from build123d import *
from OCP.BRepFilletAPI import BRepFilletAPI_MakeChamfer

# Parameters (mm, degrees)
BOSS_EXTRUDE2_DEPTH       = 40
CHAMFER1_SIZE             = 15
CHAMFER3_SIZE             = 2.5
CHAMFER3_SIZE2            = 2.68451721
M4X0_7_TAPPED_HOLE1_D     = 3.3
M4X0_7_TAPPED_HOLE1_DEPTH = 10.1
M4X0_7_TAPPED_HOLE1_TIP   = 0.991420021
SKETCH4_R                 = 11.5
CUT_EXTRUDE1_DEPTH        = 30
M6X1_0_TAPPED_HOLE1_D     = 5
M6X1_0_TAPPED_HOLE1_DEPTH = 15
M6X1_0_TAPPED_HOLE1_TIP   = 1.502151548


with BuildPart() as part:
    # Sketch1 → Boss-Extrude2 (new body)
    with BuildSketch(Plane(origin=(0, 0, 0), x_dir=(1, 0, 0), z_dir=(0, 1, 0))):
        with BuildLine():
            Line((-28, 48), (-48, 48))
            Line((-48, 48), (-93, 45))
            Line((-93, 45), (-93, -45))
            Line((-93, -45), (-48, -48))
            Line((-48, -48), (-28, -48))
            Line((-28, -48), (-28, -38.987177379))
            ThreePointArc((-28, -38.987177379), (-48, 0), (-28, 38.987177379))
            Line((-28, 38.987177379), (-28, 48))
        make_face()
    extrude(amount=BOSS_EXTRUDE2_DEPTH)

    # Chamfer1
    chamfer1_edges = [part.edges().sort_by_distance(p)[0] for p in [
        (-48, 40, 0),
    ]]
    chamfer(chamfer1_edges, length=CHAMFER1_SIZE)

    # Chamfer2
    # the kernel refuses this chamfer: 2.5 mm, written as the material it takes off along each edge
    with BuildSketch(Plane(origin=(-32.604077303, 40, -49.026394846), x_dir=(0.06649386081081782, 0.027495876610587725, 0.9974079121622642), z_dir=(-0.997785157856609, 0, 0.06651901052377412)), Plane(origin=(-108.395922697, 40, 43.973605154), x_dir=(0.06649386081081746, 0.02749587661058773, -0.9974079121622642), z_dir=(0.997785157856609, 0, 0.06651901052377378))) as chamfer2_piece_1:
        with BuildLine():
            Line((2.571682988, 0), (-0.141367887, -2.567794484))
            Line((-0.141367887, -2.567794484), (-0.191348983, -2.56641969))
            ThreePointArc((-0.191348983, -2.56641969), (-0.085323068, -1.283494574), (-0.049981096, 0.001374794))
            Line((-0.049981096, 0.001374794), (0.001374794, 0.049981096))
            ThreePointArc((0.001374794, 0.049981096), (1.286244162, 0.014639124), (2.573057782, 0.049981096))
            Line((2.573057782, 0.049981096), (2.571682988, 0))
        make_face()
    extrude(amount=75.960084991, mode=Mode.SUBTRACT)
    with BuildSketch(Plane(origin=(-93, 40, -60.430097928), x_dir=(0.9996219169112968, 0.027495876610587663, 0), z_dir=(0, 0, 1))) as chamfer2_piece_2:
        with BuildLine():
            Line((2.571682988, 0), (-0.141367887, -2.567794484))
            Line((-0.141367887, -2.567794484), (-0.191348983, -2.56641969))
            ThreePointArc((-0.191348983, -2.56641969), (-0.085323068, -1.283494574), (-0.049981096, 0.001374794))
            Line((-0.049981096, 0.001374794), (0.001374794, 0.049981096))
            ThreePointArc((0.001374794, 0.049981096), (1.286244162, 0.014639124), (2.573057782, 0.049981096))
            Line((2.573057782, 0.049981096), (2.571682988, 0))
        make_face()
    extrude(amount=120.860195856, mode=Mode.SUBTRACT)

    # Chamfer3: one chamfer whose edges measure the first distance from different faces: ONE call of the kernel's chamfer builder (chamfer() names one face for all edges)
    chamfer3_edges_1 = [part.edges().sort_by_distance(p)[0] for p in [
        (-93, 18.75, -45),
    ]]
    chamfer3_side_1 = [part.faces().sort_by_distance(p)[0] for p in [
        (-70.5, 18.75, -46.5),
    ]]
    chamfer3_edges_2 = [part.edges().sort_by_distance(p)[0] for p in [
        (-93, 18.75, 45),
    ]]
    chamfer3_side_2 = [part.faces().sort_by_distance(p)[0] for p in [
        (-93, 18.75, 0),
    ]]
    chamfer3 = BRepFilletAPI_MakeChamfer(part.part.solid().wrapped)
    for e in chamfer3_edges_1:
        chamfer3.Add(CHAMFER3_SIZE, CHAMFER3_SIZE2, e.wrapped, chamfer3_side_1[0].wrapped)  # the first distance lies on this face
    for e in chamfer3_edges_2:
        chamfer3.Add(CHAMFER3_SIZE, CHAMFER3_SIZE2, e.wrapped, chamfer3_side_2[0].wrapped)  # the first distance lies on this face
    add(Compound.cast(chamfer3.Shape()), mode=Mode.REPLACE)

    # M4x0.7 Tapped Hole1
    with Locations(Plane(origin=(-89.5, 0, 41.678571429), x_dir=(0, 0, -1), z_dir=(0, -1, 0))):
        with Locations((0, 0), (-1.410714285, 20.75), (-2.821428571, 41.5), (-2.821428571, 58), (83.357142858, 0), (84.767857143, 20.75), (86.178571429, 41.5), (86.178571429, 58), (41.678571429, 0), (41.678571429, 20), (41.678571429, 35)):
            Hole(M4X0_7_TAPPED_HOLE1_D / 2, depth=M4X0_7_TAPPED_HOLE1_DEPTH)
            with Locations((0, 0, -(M4X0_7_TAPPED_HOLE1_DEPTH + M4X0_7_TAPPED_HOLE1_TIP / 2))):  # 118° drill point
                Cone(0, M4X0_7_TAPPED_HOLE1_D / 2, M4X0_7_TAPPED_HOLE1_TIP, mode=Mode.SUBTRACT)

    # Sketch4 → Cut-Extrude1 (cut)
    with BuildSketch(Plane.ZY.offset(93)):
        with Locations((-19.907741395, 18.75)):
            Circle(SKETCH4_R)
        with Locations(Location((19.907741395, 18.75, 0), (0, 0, 180))):
            Circle(SKETCH4_R)
    extrude(amount=-CUT_EXTRUDE1_DEPTH, mode=Mode.SUBTRACT)

    # M6x1.0 Tapped Hole1
    with Locations(Plane(origin=(-78, 0, 20), x_dir=(0, 0, -1), z_dir=(0, -1, 0))):
        with Locations((0, 0), (40, 0)):
            Hole(M6X1_0_TAPPED_HOLE1_D / 2, depth=M6X1_0_TAPPED_HOLE1_DEPTH)
            with Locations((0, 0, -(M6X1_0_TAPPED_HOLE1_DEPTH + M6X1_0_TAPPED_HOLE1_TIP / 2))):  # 118° drill point
                Cone(0, M6X1_0_TAPPED_HOLE1_D / 2, M6X1_0_TAPPED_HOLE1_TIP, mode=Mode.SUBTRACT)


solid = part.part
The listing builds one solid part. Answer for the finished solid, in the listing's coordinates (mm). A direction names the side the tool comes from. Round coordinates to 2 decimals unless told otherwise and drop trailing zeros. Order: outer loops, then holes, each group sorted by start corner. A loop starts at its lowest first (then second) coordinate and runs counter-clockwise, first axis right, second up. Notation, with made-up numbers: (-1, 46.25) - (53, 46.25) arc R15 ccw to (53, 69.25) - close; hole circle Ø6 at (-4.5, 35). An arc over 180 degrees is marked (long way). Write item = value, one per line. Start each with the question number.
1) Section C-C, the plane y = 6 is taken. Count the separate pieces of the cut face and the enclosed holes in it, plus the area to 3 significant figures.
2) Section D-D, the plane y = 14 is taken. Write down the section's boundary in (x, z), plus the area to 3 significant figures.
3) For faces 1 (the flat face through (-91.7, 38.8, -0.6)), 2 (the cylindrical face through (-91.11, 5.12, 41.32)), determine the directions among +Z, -Z, +X, -X, +Y, -Y from which every point of the face is accessible in a straight line to the end or side of a thin tool.
4) Section A-A, the plane y = 18.75 is taken. Write down the section's boundary in (x, z), plus the area to 3 significant figures.
5) For a pull along Z with two mould halves and no side action, classify faces 3 (the conical face through (-89.78, 10.92, -41.62)), 4 (the flat face through (-38, 19, 48)), 5 (the flat face through (-28, 16, 44)) as released by +Z, released by -Z, zero draft, split by the parting line, or undercut.
6) Given pin 1 (14 mm diameter, centred on y = 18.75, z = -19.91, fed in from -X); pin 2 (5.5 mm diameter, centred on x = -54.5, z = 0, fed in from +Y); pin 3 (3 mm diameter, centred on y = 36, z = -7, fed in from +X), each flat-ended and moving along its own axis, determine where each tip first touches the part or whether it passes through.
7) Section B-B, the plane x = -74 is taken. Write down the section's boundary in (y, z).
8) Straight lines are drawn through the part: L1, parallel to Z at x = -84, y = 18; L2, parallel to Z at x = -89, y = 2; L3, parallel to X at y = 5, z = 44. For each, find the intervals that lie inside material, in ascending order.
Results list:
q1.separate_pieces = 1
q1.enclosed_holes = 13
q1.area = 4,870 mm^2
q2.outline = (-93, -42.32) - (-90.51, -45.17) - (-48, -48) - (-28, -48) - (-28, -38.99) arc R48 cw to (-28, 38.99) - (-28, 48) - (-48, 48) - (-90.32, 45.18) - (-93, 42.5) - (-93, 30.38) - (-63, 30.38) - (-63, 9.43) - (-93, 9.43) - (-93, -9.43) - (-63, -9.43) - (-63, -30.38) - (-93, -30.38) - close
q2.area = 3,750 mm^2
q3.face_1 = +Z, -Z, -X, +Y
q3.face_2 = -Y
q4.outline = (-93, -42.32) - (-90.51, -45.17) - (-48, -48) - (-28, -48) - (-28, -38.99) arc R48 cw to (-28, 38.99) - (-28, 48) - (-48, 48) - (-90.32, 45.18) - (-93, 42.5) - (-93, 31.41) - (-63, 31.41) - (-63, 8.41) - (-93, 8.41) - (-93, -8.41) - (-63, -8.41) - (-63, -31.41) - (-93, -31.41) - close
q4.area = 3,630 mm^2
q5.face_3 = undercut
q5.face_4 = released by +Z
q5.face_5 = zero draft
q6.pin_1 = -63
q6.pin_2 = 34.25
q6.pin_3 = -57.06
q7.outline = (0, -46.27) - (37.5, -46.27) - (40, -43.76) - (40, 43.76) - (37.5, 46.27) - (0, 46.27) - close; hole circle Ø23 at (18.75, -19.91); hole circle Ø23 at (18.75, 19.91)
q8.L1 = -45.6 to -31.38, -8.43 to 8.43, 31.38 to 45.6
q8.L2 = -45.27 to -43.25, -40.11 to -1.57, 1.57 to 40.11, 43.25 to 45.27
q8.L3 = -91.5 to -70.13, -67.37 to -49.57, -46.43 to -33.07, -29.93 to -28
